Here's the drawing with two shaded views (mm, measured from the low corner). I have some questions. Give positions to 0.01 mm unless a question says otherwise; leave off trailing zeros. Write each loop counter-clockwise with the first axis right and the second up, starting at its lowest first coordinate (ties: lowest second). Pieces come first, ordered by that corner, then holes. Notation, with made-up numbers: (25.25, -36.5) -> (38.25, -36.5) arc R34 ccw to (38.25, -4.5) -> close; hole circle Ø7 at (48, 20). An arc over 180 degrees is marked (long way). Put each result on its own line as item: value. Start each with the question number.
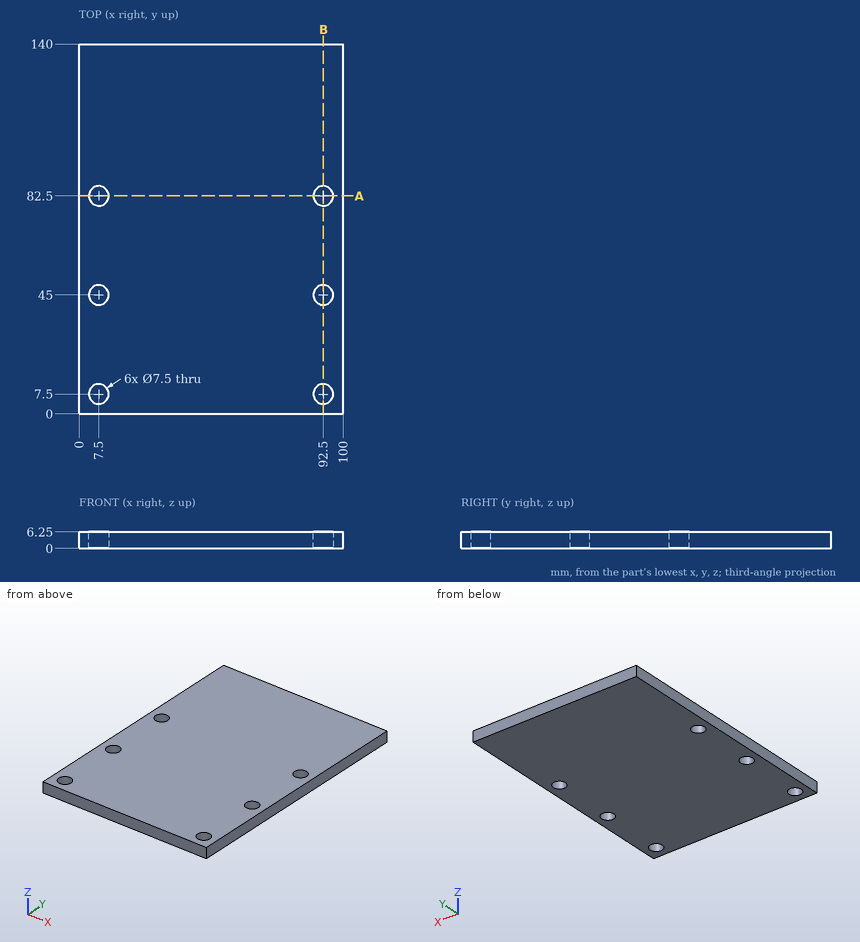
1) I need wall thicknesses on probe 1 along Y at (x, z) = (92.5, 4.75); probe 2 along Y at (x, z) = (91, 4). Which ranges of each line are inside material? Lowest first, please.
2) I want a section at B-B, the plane x = 92.5. Write out the boundary of the cut face in (y, z), and give its area (3 significant figures).
3) I'm going to push a flat-ended pin straight in: pin 1 Ø6 at (x, y) = (92.5, 45) entering from -Z. Where does the tip first touch, or does it pass through?
4) I want a section at A-A, the plane y = 82.5. Write out the boundary of the cut face in (x, z).
Established:
1. probe 1: y = 0 to 3.75, 11.25 to 41.25, 48.75 to 78.75, 86.25 to 140
1. probe 2: y = 0 to 4.06, 10.94 to 41.56, 48.44 to 79.06, 85.94 to 140
2. outline: (0, 0) -> (3.75, 0) -> (3.75, 6.25) -> (0, 6.25) -> close; (11.25, 0) -> (41.25, 0) -> (41.25, 6.25) -> (11.25, 6.25) -> close; (48.75, 0) -> (78.75, 0) -> (78.75, 6.25) -> (48.75, 6.25) -> close; (86.25, 0) -> (140, 0) -> (140, 6.25) -> (86.25, 6.25) -> close
2. area: 734 mm2
3. pin 1: passes through
4. outline: (0, 0) -> (3.75, 0) -> (3.75, 6.25) -> (0, 6.25) -> close; (11.25, 0) -> (88.75, 0) -> (88.75, 6.25) -> (11.25, 6.25) -> close; (96.25, 0) -> (100, 0) -> (100, 6.25) -> (96.25, 6.25) -> close
